For this review, take the finished solid that the model builds, in its own axes (mm). Face numbers are marked on the shaded views. A direction names the side the tool comes from. Coordinates: 2 decimals unless noted, no trailing zeros. Loops run counter-clockwise (first coordinate to the right, second up) from the corner with the lowest first, then second, coordinate; pieces in that order, holes last. Notation, with made-up numbers: (33, 68) -> (87, 68) arc R29 ccw to (87, 88) -> close; hole circle Ø5 at (-7.5, 43.25). An arc over 180 degrees is marked (long way). Answer in a Markdown table with one row per item.
from build123d import *

# Parameters (mm, degrees)
CUT_EXTRUDE1_START     = -7
CUT_EXTRUDE1_OUTLINE_R = 1.25
CUT_EXTRUDE1_DEPTH     = 7


with BuildPart() as part:
    # Sketch3 → Revolve1 (revolve)
    with BuildSketch(Plane(origin=(0, 0, 0), x_dir=(1, 0, 0), z_dir=(0, 1, 0)), mode=Mode.PRIVATE) as revolve1_sk:
        Polygon((8.717608539, 21.4), (-7.11067022, 21.4), (-7.11067022, 23.2), (-8.61067022, 23.2), (-9.61067022, 23.2), (-9.61067022, 22.2), (-8.61067022, 22.2), (-8.61067022, 18.231946605), (9.211549898, 18.231946605), (12.36932978, 13.417613419), (12.36932978, 8), (15.36932978, 8), (15.36932978, 15), (11.171491687, 21.4), align=None)
    revolve(revolve1_sk.sketch.rotate(Axis((-29.774212385, 0, 0), (1, 0, 0)), 180), axis=Axis((-29.774212385, 0, 0), (1, 0, 0)))

    # Cut-Extrude1: read off the stored shape, not the designer's step
    # Cut-Extrude1 outline → Cut-Extrude1 (cut)
    with BuildSketch(Plane(origin=(15.36932978, 0, 0), x_dir=(0, 0, -1), z_dir=(1, 0, 0)).offset(CUT_EXTRUDE1_START)):
        with BuildLine():
            add(Edge.make_bspline(
                [(-15.882949316, 9.366531964), (-19.17750573, 10.436998233), (-19.384329489, 4.195426001), (-19.591153248, -2.046146232), (-16.089773075, 3.124959731), (-12.588392902, 8.296065695), (-15.882949316, 9.366531964)],
                knots=[0, 0, 0, 2.094395102, 2.094395102, 4.188790205, 4.188790205, 6.283185307, 6.283185307, 6.283185307], degree=2, weights=[1, 0.5, 1, 0.5, 1, 0.5, 1]))
        make_face()
        with BuildLine():
            add(Edge.make_bspline(
                [(-13.816202519, -12.21116489), (-15.852350361, -15.013681966), (-9.980174473, -17.139134942), (-4.107998586, -19.264587917), (-7.944026632, -14.336617865), (-11.780054677, -9.408647813), (-13.816202519, -12.21116489)],
                knots=[0, 0, 0, 2.094395102, 2.094395102, 4.188790205, 4.188790205, 6.283185307, 6.283185307, 6.283185307], degree=2, weights=[1, 0.5, 1, 0.5, 1, 0.5, 1]))
        make_face()
        with BuildLine():
            add(Edge.make_bspline(
                [(7.344066564, -16.913446908), (9.380214406, -19.715963985), (13.216242451, -14.787993933), (17.052270496, -9.86002388), (11.180094609, -11.985476856), (5.307918722, -14.110929831), (7.344066564, -16.913446908)],
                knots=[0, 0, 0, 2.094395102, 2.094395102, 4.188790205, 4.188790205, 6.283185307, 6.283185307, 6.283185307], degree=2, weights=[1, 0.5, 1, 0.5, 1, 0.5, 1]))
        make_face()
        with BuildLine():
            add(Edge.make_bspline(
                [(18.355085271, 1.758079834), (21.649641685, 2.828546103), (18.148261512, 7.999652066), (14.646881338, 13.170758029), (14.853705097, 6.929185797), (15.060528857, 0.687613564), (18.355085271, 1.758079834)],
                knots=[0, 0, 0, 2.094395102, 2.094395102, 4.188790205, 4.188790205, 6.283185307, 6.283185307, 6.283185307], degree=2, weights=[1, 0.5, 1, 0.5, 1, 0.5, 1]))
        make_face()
        with BuildLine():
            add(Edge.make_bspline(
                [(4, 18), (4, 21.464101615), (-2, 19.732050808), (-8, 18), (-2, 16.267949192), (4, 14.535898385), (4, 18)],
                knots=[0, 0, 0, 2.094395102, 2.094395102, 4.188790205, 4.188790205, 6.283185307, 6.283185307, 6.283185307], degree=2, weights=[1, 0.5, 1, 0.5, 1, 0.5, 1]))
        make_face()
        with Locations((0, 11.5)):
            Circle(CUT_EXTRUDE1_OUTLINE_R)
        with Locations((8.131727984, 8.131727984)):
            Circle(CUT_EXTRUDE1_OUTLINE_R)
        with Locations((11.5, 0)):
            Circle(CUT_EXTRUDE1_OUTLINE_R)
        with Locations((8.131727984, -8.131727984)):
            Circle(CUT_EXTRUDE1_OUTLINE_R)
        with Locations((0, -11.5)):
            Circle(CUT_EXTRUDE1_OUTLINE_R)
        with Locations((-8.131727984, -8.131727984)):
            Circle(CUT_EXTRUDE1_OUTLINE_R)
        with Locations((-11.5, 0)):
            Circle(CUT_EXTRUDE1_OUTLINE_R)
        with Locations((-8.131727984, 8.131727984)):
            Circle(CUT_EXTRUDE1_OUTLINE_R)
    extrude(amount=CUT_EXTRUDE1_DEPTH, mode=Mode.SUBTRACT)


solid = part.part
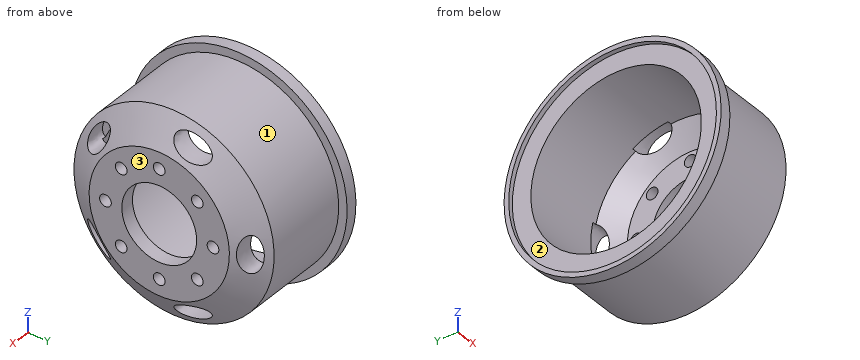
Item 1: For the marked faces 1, 2 and 3, list the 3-axis set-ups (+Z, -Z, +X, -X, +Y, -Y) from which the entire face can be reached by the end or side of a thin tool; tool diameter is ignored.
Worked answers:
| item | result |
|---|---|
| face 1 | +X |
| face 2 | -X |
| face 3 | +Z, -Z, +X, +Y, -Y |
Item 2: For L1, parallel to Y at x = 11.5, z = 9.5; L2, parallel to Y at x = 14.65, z = 0; L3, parallel to X at y = -12, z = -1.5, list the stretches that pass through material, from the lowest coordinate up.
Worked answers:
| item | result |
|---|---|
| L1 | -18.62 to -17.29, -12.88 to -11.27, 11.27 to 18.62 |
| L2 | -16.1 to -12.75, -10.25 to -8, 8 to 10.25, 12.75 to 16 |
| L3 | 12.37 to 15.37 |
Item 3: Take a section at B-B, the plane x = -5.5. State the section outline as (y, z) points, and give its area (3 significant figures).
Worked answers:
| item | result |
|---|---|
| outline | circle Ø42.8 at (0, 0); hole circle Ø36.46 at (0, 0) |
| area | 394 mm² |
Item 4: Take a section at A-A, the plane y = 0. Count the separate pieces of the cut face and the enclosed holes in it, and give its area (3 significant figures).
Worked answers:
| item | result |
|---|---|
| separate pieces | 4 |
| enclosed holes | 0 |
| area | 194 mm² |
Item 5: Insertion check: pin 1 (4 mm diameter, centred on y = 0, z = -11.5, fed in from -X); pin 2 (3 mm diameter, centred on y = -13, z = 15.5, fed in from -X); pin 3 (6 mm diameter, centred on y = -1, z = -18, fed in from +X). Each pin has a flat end and moves straight along its axis. Give the tip position at first contact, or say it passes through.
Worked answers:
| item | result |
|---|---|
| pin 1 | x = 12.32 |
| pin 2 | x = -8.61 |
| pin 3 | x = 15.35 |
